```python
from build123d import *

# Parameters (mm, degrees)
SKETCH1_R           = 2.1
BOSS_EXTRUDE1_DEPTH = 2.5


with BuildPart() as part:
    # Sketch1 → Boss-Extrude1 (new body)
    with BuildSketch(Plane(origin=(0, 0, 0), x_dir=(1, 0, 0), z_dir=(0, 1, 0))):
        with BuildLine():
            Line((4, -36), (4, -40))
            ThreePointArc((4, -40), (0, -44), (-4, -40))
            Line((-4, -40), (-4, -32))
            Line((-4, -32), (-4, -20.894729077))
            ThreePointArc((-4, -20.894729077), (11.843809939, 1.649089261), (13.171572875, 29.171572875))
            ThreePointArc((13.171572875, 29.171572875), (12, 32), (13.171572875, 34.828427125))
            Line((13.171572875, 34.828427125), (21.171572875, 42.828427125))
            ThreePointArc((21.171572875, 42.828427125), (26.828427125, 42.828427125), (26.828427125, 37.171572875))
            Line((26.828427125, 37.171572875), (22.828427125, 33.171572875))
            ThreePointArc((22.828427125, 33.171572875), (21.232537081, 0.397959844), (4, -27.525081572))
            Line((4, -27.525081572), (4, -36))
        make_face()
        with Locations(Location((0, -32, 0), (0, 0, 270))):
            Circle(SKETCH1_R, mode=Mode.SUBTRACT)
        with Locations(Location((0, -40, 0), (0, 0, 270))):
            Circle(SKETCH1_R, mode=Mode.SUBTRACT)
        with Locations(Location((16, 32, 0), (0, 0, 270))):
            Circle(SKETCH1_R, mode=Mode.SUBTRACT)
        with Locations(Location((24, 40, 0), (0, 0, 270))):
            Circle(SKETCH1_R, mode=Mode.SUBTRACT)
        with Locations(Location((16, 0, 0), (0, 0, 270))):
            Circle(SKETCH1_R, mode=Mode.SUBTRACT)
    extrude(amount=BOSS_EXTRUDE1_DEPTH)


solid = part.part
```
The listing builds one solid part. Answer for the finished solid, in the listing's coordinates (mm). A direction names the side the tool comes from. Round coordinates to 2 decimals unless told otherwise and drop trailing zeros. Loops run counter-clockwise (first coordinate to the right, second up) from the corner with the lowest first, then second, coordinate; pieces in that order, holes last.
1) Given P1, Ø1, axis at y = 2, z = 30.5, coming from the +X side, flat-ended and moving along its own axis, determine where the tip first touches the part or whether it passes through.
Outcome:
P1: stops at x = 4
2) A cutting plane is placed at A-A on z = 32. Determine the outline of the cut face in (x, y), plus the area to 3 significant figures.
Outcome:
outline: (-4, 0) - (-2.1, 0) - (-2.1, 2.5) - (-4, 2.5) - close; (2.1, 0) - (4, 0) - (4, 2.5) - (2.1, 2.5) - close
area: 9.50 mm2
3) A cutting plane is placed at C-C on x = 0. Determine the outline of the cut face in (y, z).
Outcome:
outline: (0, 17.31) - (2.5, 17.31) - (2.5, 29.9) - (0, 29.9) - close; (0, 34.1) - (2.5, 34.1) - (2.5, 37.9) - (0, 37.9) - close; (0, 42.1) - (2.5, 42.1) - (2.5, 44) - (0, 44) - close
4) For faces 4 (the face through (24.856, 1.232, -35.2)), 5 (the face through (17.116, 1.232, -38.772)), 6 (the face through (4, 1, 34)), determine the directions among +Z, -Z, +X, -X, +Y, -Y from which every point of the face is accessible in a straight line to the end or side of a thin tool.
Outcome:
face 4: +X, +Y, -Y
face 5: -Z, -X, +Y, -Y
face 6: +Z, +X, +Y, -Y
5) Consider line 1 (X direction, y = 1.35, z = 32); line 2 (Z direction, x = 15.5, y = 2.2); line 3 (Z direction, x = 17, y = 1.2). Determine where each line is inside the solid, lowest interval first.
Outcome:
line 1: x = -4 to -2.1, 2.1 to 4
line 2: z = -37.16 to -34.04, -29.96 to -2.04, 2.04 to 12.78
line 3: z = -38.66 to -33.85, -30.15 to -1.85, 1.85 to 10.01
6) A cutting plane is placed at B-B on y = 1.1. Determine the outline of the cut face in (x, z).
Outcome:
outline: (-4, 20.89) arc R49.48 cw to (13.17, -29.17) arc R4 ccw to (13.17, -34.83) - (21.17, -42.83) arc R4 ccw to (26.83, -37.17) - (22.83, -33.17) arc R65.76 ccw to (4, 27.53) - (4, 40) arc R4 ccw to (-4, 40) - close; hole circle Ø4.2 at (0, 32); hole circle Ø4.2 at (0, 40); hole circle Ø4.2 at (16, -32); hole circle Ø4.2 at (16, 0); hole circle Ø4.2 at (24, -40)
7) For a pull along Z with two mould halves and no side action, classify faces 1 (the face through (13, 0, -3)), 2 (the face through (0.09, 1.23, 37.9)), 3 (the face through (0, 1, 44)) as released by +Z, released by -Z, zero draft, split by the parting line, or undercut.
Outcome:
face 1: zero draft
face 2: undercut
face 3: released by +Z
8) A cutting plane is placed at D-D on x = 25. Determine the outline of the cut face in (y, z), plus the area to 3 significant figures.
Outcome:
outline: (0, -43.87) - (2.5, -43.87) - (2.5, -41.85) - (0, -41.85) - close; (0, -38.15) - (2.5, -38.15) - (2.5, -35.34) - (0, -35.34) - close
area: 12.1 mm2
